Geometry: final body of the model. Coordinates: model frame, mm. A direction names the side the tool comes from. Give positions to 0.01 mm unless a question says otherwise; leave off trailing zeros. Write each loop counter-clockwise with the first axis right and the second up, starting at its lowest first coordinate (ties: lowest second). Pieces come first, ordered by that corner, then holes. Notation, with made-up numbers: M -6.75,73.5 L 29.25,73.5 A11 cw 29.25,85.5 Z; hole C -22.75,81 d4. An arc over 180 degrees is marked long. Use one line per item in the form item = value. Start each with the question number.
Item 1: Material intervals for line 1 along X through (y, z) = (4.2, 0); line 2 along Y through (x, z) = (7.25, -7); line 3 along Z through (x, y) = (0, 2.9), sorted ascending. Write a range as from..to.
Item 2: Section query A-A on z = 0. Return loops of the section in (x, y), then the cut area to 3 significant figures.
Item 3: Section query B-B on x = 0. Return loops of the section in (y, z), then the cut area to 4 significant figures.
Item 4: Access query for faces 1 (the flat face through (-0.5, 4, 10)), 2 (the cylindrical face through (0, 6, -10)), 3 (the cylindrical face through (-2.49, 0.49, 9.71)). Directions: +Z, -Z, +X, -X, +Y, -Y. A direction counts if a zero-diameter tool reaches every point of the face in a straight line with its end or side. Return the directions, or none.
Item 5: Section query D-D on y = 5.75. Return loops of the section in (x, z).
Item 6: Section query C-C on y = 3.5. Return loops of the section in (x, z), then the cut area to 3 significant figures.
Item 7: Contact query for flat-ended pins moving along their axis: P1, Ø2, axis at x = -4.5, z = 7, coming from the +Y side; P2, Ø2, axis at y = 1, z = -9, coming from the -X side; P3, Ø1, axis at x = -5.5, y = 2.5, coming from the -Z side. Output: stop coordinate, or through.
from build123d import *

# Parameters (mm, degrees)
SKETCH1_R           = 11.25
SKETCH1_R_2         = 8.5
BOSS_EXTRUDE1_DEPTH = 6.4
SKETCH2_R           = 10
CUT_EXTRUDE1_DEPTH  = 1
CHAMFER1_SIZE       = 0.5
SKETCH3_R           = 2.5
CUT_EXTRUDE2_DEPTH  = 1
SKETCH4_W           = 1
SKETCH4_H           = 7.023795273
CUT_EXTRUDE3_DEPTH  = 10


with BuildPart() as part:
    # Sketch1 → Boss-Extrude1 (new body)
    with BuildSketch(Plane(origin=(0, 0, 0), x_dir=(1, 0, 0), z_dir=(0, 1, 0))):
        with Locations(Location((0, 0, 0), (0, 0, 270))):
            Circle(SKETCH1_R)
        with Locations(Location((0, 0, 0), (0, 0, 270))):
            Circle(SKETCH1_R_2, mode=Mode.SUBTRACT)
    extrude(amount=BOSS_EXTRUDE1_DEPTH)

    # Sketch2 → Cut-Extrude1 (cut)
    with BuildSketch(Plane(origin=(0, 6.4, 0), x_dir=(1, 0, 0), z_dir=(0, 1, 0))):
        with Locations(Location((0, 0, 0), (0, 0, 270))):
            Circle(SKETCH2_R)
    extrude(amount=-CUT_EXTRUDE1_DEPTH, mode=Mode.SUBTRACT)

    # Chamfer1
    chamfer1_edges = [part.edges().sort_by_distance(p)[0] for p in [
        (0, 0, -11.25),
        (0, 0, -8.5),
    ]]
    chamfer(chamfer1_edges, length=CHAMFER1_SIZE)

    # Sketch3 → Cut-Extrude2 (cut)
    with BuildSketch(Plane.XZ):
        with Locations((0, 9.5)):
            Circle(SKETCH3_R)
        with Locations((8.227241336, -4.75)):
            Circle(SKETCH3_R)
        with Locations((-8.227241336, -4.75)):
            Circle(SKETCH3_R)
    extrude(amount=-CUT_EXTRUDE2_DEPTH, mode=Mode.SUBTRACT)

    # Sketch4 → Cut-Extrude3 (cut)
    with BuildSketch(Plane.XZ):
        with Locations((0, 9.698212769)):
            Rectangle(SKETCH4_W, SKETCH4_H)
    extrude(amount=-CUT_EXTRUDE3_DEPTH, mode=Mode.SUBTRACT)


solid = part.part
Answer sheet:
q1.line_1 = -11.25..-8.5, 8.5..11.25
q1.line_2 = 1..6.4
q1.line_3 = -11.25..-8.5
q2.outline = M -11.25,0.5 L -10.75,0 L -9,0 L -8.5,0.5 L -8.5,5.4 L -10,5.4 L -10,6.4 L -11.25,6.4 Z; M 8.5,0.5 L 9,0 L 10.75,0 L 11.25,0.5 L 11.25,6.4 L 10,6.4 L 10,5.4 L 8.5,5.4 Z
q2.area = 31.7 mm2
q3.outline = M 0,-10.75 L 0.5,-11.25 L 6.4,-11.25 L 6.4,-10 L 5.4,-10 L 5.4,-8.5 L 0.5,-8.5 L 0,-9 Z
q3.area = 15.85 mm2
q4.face_1 = +Z, +Y, -Y
q4.face_2 = +Y
q4.face_3 = -Y
q5.outline = M -0.5,9.99 L -0.5,11.24 A11.25 ccw long 0.5,11.24 L 0.5,9.99 A10 cw long Z
q6.outline = M -0.5,8.49 L -0.5,11.24 A11.25 ccw long 0.5,11.24 L 0.5,8.49 A8.5 cw long Z
q6.area = 168 mm2
q7.P1 = 5.4
q7.P2 = -7.91
q7.P3 = -10.08
